Design review of the part built by this model. Coordinates are the model's own, in mm. Face numbers are marked on the shaded views. A direction names the side the tool comes from. Give positions to 0.01 mm unless a question says otherwise; leave off trailing zeros. Order: outer loops, then holes, each group sorted by start corner. A loop starts at its lowest first (then second) coordinate and runs counter-clockwise, first axis right, second up. Notation, with made-up numbers: (-20.5, 88) -> (-15.5, 88) arc R18 cw to (-15.5, 95) -> close; hole circle Ø10 at (-23, 1.25). An arc over 180 degrees is marked (long way). Return JSON: item names as keys, results as strings.
Autodesk Inventor part; units mm, degrees
ref_plane "YZ Plane" through (0, 0, 0) normal (1, 0, 0) x (0, 1, 0)
ref_plane "XZ Plane" through (0, 0, 0) normal (0, 1, 0) x (-1, 0, 0)
ref_plane "XY Plane" through (0, 0, 0) normal (0, 0, 1) x (1, 0, 0)
sketch "Skizze1" plane through (0, 0, 0) normal (1, 0, 0) x (0, 1, 0)
  line L0 (0, 0) -> (-10, 0) construction
  circle A0 centre (0, 0) radius 1.1
  circle A1 centre (-10, 0) radius 1.1
  arc A2 (-10, 2.5) -> (-10, -2.5) centre (-10, 0) ccw
  line L1 (-10, -2.5) -> (2, -2.5)
  line L2 (-10, 2.5) -> (-0.5, 2.5)
  arc A3 (2, 0) -> (-0.5, 2.5) centre (-0.5, 0) ccw
  line L3 (2, 0) -> (2, -2.5)
  dimension "d0" = 10
  dimension "d1" = 2.2
  dimension "d2" = 2.2
  dimension "d3" = 2.5
  dimension "d8" = 2.5
  dimension "d9" = 2
extrude "Extrusion1" add sketch "Skizze1" along normal mid plane 4
chamfer "Fase1" distance 0.5 angle 45 10 edges at (2, 1.2678, 1.7678) (2, -5.25, 2.5) (2, -12.5, 0) (2, -4, -2.5) (2, 2, -1.25) (-2, 1.2678, 1.7678) (-2, -5.25, 2.5) (-2, -12.5, 0) (-2, -4, -2.5) (-2, 2, -1.25)
sketch "Skizze5" plane through (-1.5, -10, 2.5) normal (0, 0, 1) x (1, 0, 0)
  line L0 (1.5, 14.9) -> (1.5, -5.4)
  line L1 (-1.3, 10) -> (4.3, 10)
  line L2 (3.5, 8) -> (-0.5, 8)
  line L3 (-0.5, 8) -> (-0.5, 7)
  line L4 (-0.5, 7) -> (3.5, 7)
  line L5 (3.5, 7) -> (3.5, 8)
  line L6 (3.5, 0) -> (3.5, 9.5)
  line L7 (-0.5, 9.5) -> (-0.5, 0)
  point P0 (1.5, 10)
  dimension "d26" = 1
  dimension "d27" = 2
extrude "Extrusion4" cut sketch "Skizze5" against normal blind 1
pattern_linear "Rechteckige Anordnung1" [suppressed]
equation "\"d2\" = d1"
properties part number "Chipanschlag L2.0"
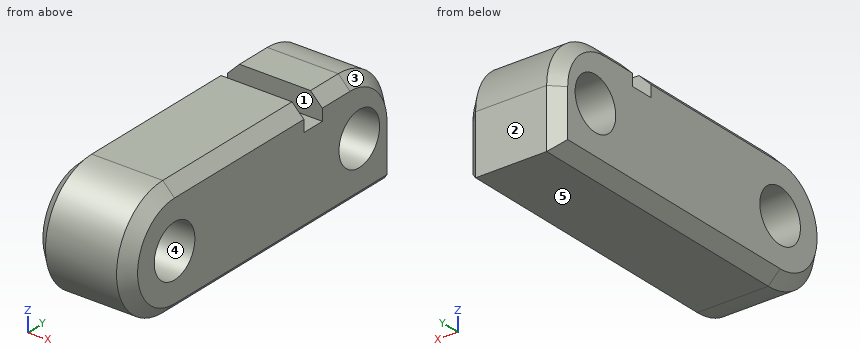
Item 1: Machinability: for the marked faces 1 and 2, which of the approach directions +Z, -Z, +X, -X, +Y, -Y give a long, thin tool a straight path to every point of the face, cutting with its end or side? Answer none if there is none.
Result set:
{"face 1": "+Z, +X, -X", "face 2": "+Z, -Z, +X, -X, +Y"}
Item 2: Add section C-C (z = -0.45). Give the number of separate pieces and of enclosed holes in the cut face, plus the area to 3 significant figures.
Result set:
{"separate pieces": "3", "enclosed holes": "0", "area": "41.3 mm^2"}
Item 3: For pin 1 (2 mm diameter, centred on x = 0.5, z = 0.5, fed in from -Y); pin 2 (0.8 mm diameter, centred on x = 0, z = 2, fed in from -Y); pin 3 (1.1 mm diameter, centred on x = 1, z = 2, fed in from +Y), all flat-tipped, find the tip position at first contact; note any pin that passes through.
Result set:
{"pin 1": "stops at y = -12.5", "pin 2": "stops at y = -11.92", "pin 3": "stops at y = 1.54"}
Item 4: Add section B-B (y = -4). Give the boundary of the cut face in (x, z).
Result set:
{"outline": "(-2, -2) -> (-1.5, -2.5) -> (1.5, -2.5) -> (2, -2) -> (2, 2) -> (1.5, 2.5) -> (-1.5, 2.5) -> (-2, 2) -> close"}
Item 5: Wall thickness on L1, parallel to Z at x = 1.2, y = -10; L2, parallel to Y at x = 1.2, z = -0.6; L3, parallel to Z at x = 1.15, y = 0: over which ranges is each line inside the solid? List them lowest first. Write a range as [from, to].
Result set:
{"L1": "z = [-2.5, -1.1], [1.1, 2.5]", "L2": "y = [-12.43, -10.92], [-9.08, -0.92], [0.92, 2]", "L3": "z = [-2.5, -1.1], [1.1, 2.45]"}
Item 6: Mouldability with a two-part tool opening along Z and no side actions: class the marked faces 3, 4 and 5 as released by +Z, released by -Z, zero draft, split by the parting line, or undercut.
Result set:
{"face 3": "released by +Z", "face 4": "undercut", "face 5": "released by -Z"}
Item 7: Add section A-A (x = 1.2). Give the boundary of the cut face in (y, z), plus the area to 3 significant figures.
Result set:
{"outline": "(-10, -2.5) -> (2, -2.5) -> (2, 0) arc R2.5 ccw to (-0.5, 2.5) -> (-2, 2.5) -> (-2, 1.5) -> (-3, 1.5) -> (-3, 2.5) -> (-10, 2.5) arc R2.5 ccw to start; hole circle Ø2.2 at (-10, 0); hole circle Ø2.2 at (0, 0)", "area": "59.9 mm^2"}
